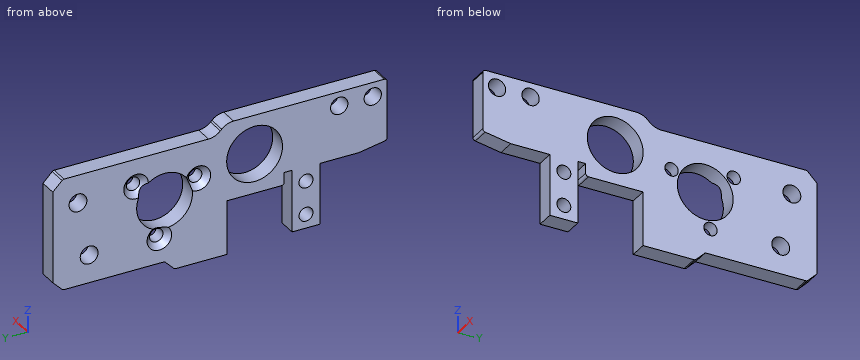
```python
from build123d import *

# Parameters (mm, degrees)
SKETCH1_R                                       = 5
SKETCH1_R_2                                     = 1.6
SKETCH1_R_3                                     = 1.25
SKETCH1_R_4                                     = 1.55
BOSS_EXTRUDE1_DEPTH                             = 3.18
CHAMFER1_SIZE                                   = 5
CHAMFER1_SIZE2                                  = 0.881634904
CSK_FOR_M2_FLAT_HEAD_MACHINE_SCREW1_D           = 2.4
CSK_FOR_M2_FLAT_HEAD_MACHINE_SCREW1_DEPTH       = 3.508967257
CSK_FOR_M2_FLAT_HEAD_MACHINE_SCREW1_CSINK_D     = 4.4
CSK_FOR_M2_FLAT_HEAD_MACHINE_SCREW1_CSINK_ANGLE = 90
CSK_FOR_M2_FLAT_HEAD_MACHINE_SCREW1_TIP         = 0.721032743
SKETCH3_R                                       = 5
CUT_EXTRUDE4_DEPTH                              = 65.449891389
FILLET2_R                                       = 3
CHAMFER2_SIZE                                   = 1.8
FILLET4_R                                       = 0.5


with BuildPart() as part:
    # Sketch1 → Boss-Extrude1 (new body)
    with BuildSketch(Plane(origin=(0, 0, 0), x_dir=(0, 0, -1), z_dir=(1, 0, 0))):
        Polygon((0, 0), (0, 28.7), (2, 30.7), (2, 59.81), (22, 59.81), (22, 39.81), (23.8, 39.81), (23.8, 28.68), (14.1, 28.68), (14.1, 18.4), (11.85, 18.4), (11.85, 17), (23, 17), (23, 12), (12, 12), (12, 0), align=None)
        with Locations(Location((7, 23.7, 0), (0, 0, 180))):
            Circle(SKETCH1_R, mode=Mode.SUBTRACT)
        with Locations(Location((7, 55.31, 0), (0, 0, 180))):
            Circle(SKETCH1_R_2, mode=Mode.SUBTRACT)
        with Locations(Location((17, 53.31, 0), (0, 0, 180))):
            Circle(SKETCH1_R_2, mode=Mode.SUBTRACT)
        with Locations(Location((20.5, 14.5, 0), (0, 0, 180))):
            Circle(SKETCH1_R_3, mode=Mode.SUBTRACT)
        with Locations(Location((14.5, 14.5, 0), (0, 0, 180))):
            Circle(SKETCH1_R_3, mode=Mode.SUBTRACT)
        with Locations(Location((2.55, 2.55, 0), (0, 0, 180))):
            Circle(SKETCH1_R_4, mode=Mode.SUBTRACT)
        with Locations(Location((2.55, 8.55, 0), (0, 0, 180))):
            Circle(SKETCH1_R_4, mode=Mode.SUBTRACT)
    extrude(amount=BOSS_EXTRUDE1_DEPTH)

    # Chamfer1
    chamfer1_edges = [part.edges().sort_by_distance(p)[0] for p in [
        (1.59, 0, -12),
    ]]
    chamfer1_side = [part.faces().sort_by_distance(p)[0] for p in [
        (1.59, 6, -12),
    ]]
    chamfer(chamfer1_edges, length=CHAMFER1_SIZE, length2=CHAMFER1_SIZE2, reference=chamfer1_side[0])

    # CSK for M2 Flat Head Machine Screw1
    with Locations(Plane.ZY):
        with Locations((-6.974936087, 44.914674329), (-17.432559713, 40.744769284), (-8.592504199, 33.773154083)):
            CounterSinkHole(CSK_FOR_M2_FLAT_HEAD_MACHINE_SCREW1_D / 2, CSK_FOR_M2_FLAT_HEAD_MACHINE_SCREW1_CSINK_D / 2, depth=CSK_FOR_M2_FLAT_HEAD_MACHINE_SCREW1_DEPTH, counter_sink_angle=CSK_FOR_M2_FLAT_HEAD_MACHINE_SCREW1_CSINK_ANGLE)
            with Locations((0, 0, -(CSK_FOR_M2_FLAT_HEAD_MACHINE_SCREW1_DEPTH + CSK_FOR_M2_FLAT_HEAD_MACHINE_SCREW1_TIP / 2))):  # 118° drill point
                Cone(0, CSK_FOR_M2_FLAT_HEAD_MACHINE_SCREW1_D / 2, CSK_FOR_M2_FLAT_HEAD_MACHINE_SCREW1_TIP, mode=Mode.SUBTRACT)

    # Sketch3 → Cut-Extrude4 (cut, through all)
    with BuildSketch(Plane.ZY):
        with Locations((-11, 39.810865899)):
            Circle(SKETCH3_R)
    extrude(amount=-CUT_EXTRUDE4_DEPTH, mode=Mode.SUBTRACT)

    # Fillet2
    fillet2_edges = [part.edges().sort_by_distance(p)[0] for p in [
        (1.59, 28.7, 0),
        (1.59, 30.7, -2),
    ]]
    fillet(fillet2_edges, radius=FILLET2_R)

    # Chamfer2
    chamfer2_edges = [part.edges().sort_by_distance(p)[0] for p in [
        (1.59, 59.81, -22),
        (1.59, 59.81, -2),
        (1.59, 39.81, -23.8),
    ]]
    chamfer(chamfer2_edges, length=CHAMFER2_SIZE - 0.0001)  # a hair under: the kernel refuses the full size

    # Fillet4
    fillet4_edges = [part.edges().sort_by_distance(p)[0] for p in [
        (1.59, 38.0101, -23.8),
        (1.59, 58.0101, -22),
        (1.59, 58.0101, -2),
        (1.59, 0, 0),
        (1.59, 18.4, -14.1),
        (1.59, 0, -11.118365096),
    ]]
    fillet(fillet4_edges, radius=FILLET4_R)


solid = part.part
```
Model file for the job. Use its own axes, mm. Round coordinates to 2 decimals unless told otherwise and drop trailing zeros. Order: outer loops, then holes, each group sorted by start corner. A loop starts at its lowest first (then second) coordinate and runs counter-clockwise, first axis right, second up. Notation, with made-up numbers: M 63,-10 L 74,-10 A16 ccw 74,19 Z; hole C 5.25,-20 d5. An arc over 180 degrees is marked long. Use CSV: the item, a comma, the result in double quotes.
Item 1: Saw through at C-C (z = -17). State how many separate pieces and enclosed holes the cut face has, plus the area to 3 significant figures.
Worked answers:
separate pieces,"4"
enclosed holes,"0"
area,"96.6 mm²"
Item 2: Probe probe 1 along Z at (x, y) = (1.15, 14.5); probe 2 along Y at (x, z) = (1.35, -2.55); probe 3 along Y at (x, z) = (0.85, -17). List the from-to ranges inside material, lowest first.
Worked answers:
probe 1,"-23 to -21.75, -19.25 to -15.75, -13.25 to 0"
probe 2,"0 to 1, 4.1 to 7, 10.1 to 21.42, 25.98 to 58.56"
probe 3,"12 to 17, 28.68 to 39.47, 42.02 to 51.71, 54.91 to 59.81"
Item 3: Saw through at A-A (y = 23.7). List the corners of the cut face in (x, z).
Worked answers:
outline,"M 0,-14.1 L 3.18,-14.1 L 3.18,-12 L 0,-12 Z; M 0,-2 L 3.18,-2 L 3.18,0 L 0,0 Z"
Item 4: Saw through at B-B (y = 2.55). List the corners of the cut face in (x, z).
Worked answers:
outline,"M 0,-11.57 L 3.18,-11.57 L 3.18,-4.1 L 0,-4.1 Z; M 0,-1 L 3.18,-1 L 3.18,0 L 0,0 Z"
Item 5: Pin check, flat tips, straight feed: pin 1 (1 mm diameter, centred on x = 2.5, y = 13.5, fed in from -Z); pin 2 (3 mm diameter, centred on y = 44.91, z = -6.97, fed in from -X); pin 3 (1.6 mm diameter, centred on x = 2, y = 8, fed in from -Z); pin 4 (4 mm diameter, centred on y = 26, z = -6, fed in from -X). Stop position of each tip, or through.
Worked answers:
pin 1,"z = -23"
pin 2,"x = 0.69"
pin 3,"z = -12"
pin 4,"through"
